```python
from build123d import *

# Parameters (mm, degrees)
SKETCH1_7_R         = 27.5
BOSS_EXTRUDE1_DEPTH = 3.5
CUT_EXTRUDE8_REACH  = 44.335
SKETCH4_R           = 6


with BuildPart() as part:
    # Sketch1 → Revolve16 (revolve)
    with BuildSketch(Plane.XY, mode=Mode.PRIVATE) as revolve16_sk:
        with BuildLine():
            Line((-9.25, 22.000000003), (-9.25, 27.485223303))
            ThreePointArc((-9.25, 27.485223303), (0, 29), (9.25, 27.485223303))
            Line((9.25, 27.485223303), (9.25, 22.000000003))
            Line((9.25, 22.000000003), (-9.25, 22.000000003))
        make_face()
    revolve(revolve16_sk.sketch.rotate(Axis((-9.25, 22.000000003, 0), (1, 0, 0)), 180), axis=Axis((-9.25, 22.000000003, 0), (1, 0, 0)))



with BuildPart() as body_2:
    # Sketch1_3 → Revolve17 (revolve)
    with BuildSketch(Plane.XY, mode=Mode.PRIVATE) as revolve17_sk:
        with BuildLine():
            Line((-18.064836163, 15.595646653), (-23.281593526, 17.29067387))
            ThreePointArc((-23.281593526, 17.29067387), (-27.580638973, 8.961492837), (-28.998407922, -0.303871681))
            Line((-28.998407922, -0.303871681), (-23.781650559, -1.998898899))
            Line((-23.781650559, -1.998898899), (-18.064836163, 15.595646653))
        make_face()
    revolve(revolve17_sk.sketch.rotate(Axis((-23.781650559, -1.998898899, 0), (0.3090169943749582, 0.9510565162951501, 0)), 180), axis=Axis((-23.781650559, -1.998898899, 0), (0.3090169943749582, 0.9510565162951501, 0)))


with BuildPart() as body_3:
    # Sketch1_4 → Revolve18 (revolve)
    with BuildSketch(Plane.XY, mode=Mode.PRIVATE) as revolve18_sk:
        with BuildLine():
            Line((-20.41468275, -12.361360295), (-23.638816111, -16.798999162))
            ThreePointArc((-23.638816111, -16.798999162), (-17.045772316, -23.461492837), (-8.672001715, -27.67302633))
            Line((-8.672001715, -27.67302633), (-5.447868354, -23.235387462))
            Line((-5.447868354, -23.235387462), (-20.41468275, -12.361360295))
        make_face()
    revolve(revolve18_sk.sketch.rotate(Axis((-5.447868354, -23.235387462, 0), (-0.8090169943749421, 0.5877852522924805, 0)), 180), axis=Axis((-5.447868354, -23.235387462, 0), (-0.8090169943749421, 0.5877852522924805, 0)))


with BuildPart() as body_4:
    # Sketch1_5 → Revolve19 (revolve)
    with BuildSketch(Plane.XY, mode=Mode.PRIVATE) as revolve19_sk:
        with BuildLine():
            Line((5.447868354, -23.235387462), (8.672001715, -27.67302633))
            ThreePointArc((8.672001715, -27.67302633), (17.045772316, -23.461492837), (23.638816111, -16.798999162))
            Line((23.638816111, -16.798999162), (20.41468275, -12.361360295))
            Line((20.41468275, -12.361360295), (5.447868354, -23.235387462))
        make_face()
    revolve(revolve19_sk.sketch.rotate(Axis((20.41468275, -12.361360295, 0), (-0.8090169943749509, -0.5877852522924685, 0)), 180), axis=Axis((20.41468275, -12.361360295, 0), (-0.8090169943749509, -0.5877852522924685, 0)))


with BuildPart() as body_5:
    # Sketch1_6 → Revolve20 (revolve)
    with BuildSketch(Plane.XY, mode=Mode.PRIVATE) as revolve20_sk:
        with BuildLine():
            Line((23.781650559, -1.998898899), (28.998407922, -0.303871681))
            ThreePointArc((28.998407922, -0.303871681), (27.580638973, 8.961492837), (23.281593526, 17.29067387))
            Line((23.281593526, 17.29067387), (18.064836163, 15.595646653))
            Line((18.064836163, 15.595646653), (23.781650559, -1.998898899))
        make_face()
    revolve(revolve20_sk.sketch.rotate(Axis((18.064836163, 15.595646653, 0), (0.30901699437494456, -0.9510565162951546, 0)), 180), axis=Axis((18.064836163, 15.595646653, 0), (0.30901699437494456, -0.9510565162951546, 0)))


with BuildPart() as part_1:
    add(part.part)

    add(body_2.part)  # Boss-Extrude1 merges body 2

    add(body_3.part)  # Boss-Extrude1 merges body 3

    add(body_4.part)  # Boss-Extrude1 merges body 4

    add(body_5.part)  # Boss-Extrude1 merges body 5
    # Sketch1_7 → Boss-Extrude1 (add, symmetric)
    with BuildSketch(Plane.XY):
        Circle(SKETCH1_7_R)
    extrude(amount=BOSS_EXTRUDE1_DEPTH, both=True)

    # Sketch4 → Cut-Extrude8 (cut, up to next)
    with BuildSketch(Plane(origin=(0, 0, -3.5), x_dir=(-1, 0, 0), z_dir=(0, 0, -1)), mode=Mode.PRIVATE) as cut_extrude8_sk1:
        Circle(SKETCH4_R)
    cut_extrude8_tool1 = extrude(cut_extrude8_sk1.sketch, amount=-CUT_EXTRUDE8_REACH, mode=Mode.PRIVATE) & part_1.part
    add(cut_extrude8_tool1.solids().sort_by_distance((0, 0, -3.5))[0], mode=Mode.SUBTRACT)


solid = part_1.part
```
Check sheet for the modelled part. Datum: model origin and axes. Units: mm. A direction names the side the tool comes from. Round coordinates to 2 decimals unless told otherwise and drop trailing zeros. Order: outer loops, then holes, each group sorted by start corner. A loop starts at its lowest first (then second) coordinate and runs counter-clockwise, first axis right, second up. Notation, with made-up numbers: (-18.75, -39.75) -> (8.25, -39.75) arc R30 ccw to (8.25, -14.75) -> close; hole circle Ø4 at (-26.5, 4). An arc over 180 degrees is marked (long way). Use CSV: the item, a comma, the result in double quotes.
(1) Material ranges on line 1 along Y through (x, z) = (-8, 4); line 2 along X through (y, z) = (-13, -4.75); line 3 along Z through (x, y) = (4, 10.5), recorded low to high. Write a range as from..to.
Worked out:
line 1,"-26.21..-14.38, 17.7..26.3"
line 2,"-20.88..-10.84, 10.84..20.88"
line 3,"-3.5..3.5"
(2) Draft check along X on faces 6 (the face through (27.78, -0.7, -0.03)), 7 (the face through (-22.063, 16.895, -0.026)), 8 (the face through (-6.5, -0.4, -3.5)), 9 (the face through (-26.19, -8.39, 0.05)). Enter one of: pulls with the +X half, pulls with the -X half, needs draft (parallel to the pull), parting line crosses it, or undercut.
Worked out:
face 6,"pulls with the +X half"
face 7,"undercut"
face 8,"undercut"
face 9,"pulls with the -X half"
(3) Depth check by flat-ended pin: pin 1 (6 mm diameter, centred on y = -20, z = -2, fed in from +X); pin 2 (8 mm diameter, centred on x = -23, y = 19, fed in from +Z); pin 3 (4 mm diameter, centred on x = 4.5, y = -10, fed in from -Z). Enter the tip coordinate at first touch or a pass-through.
Worked out:
pin 1,"x = 23.27"
pin 2,"z = 5.11"
pin 3,"z = -3.5"
(4) Tool access check on faces 1 (the face through (-22.886, -15.762, -0.026)), 2 (the face through (7.92, -26.64, -0.03)), 3 (the face through (-6.5, -0.4, 3.5)), 4 (the face through (-9.25, 26.2, 0)), 5 (the face through (9.25, 23, 4)). Record the directions out of +Z, -Z, +X, -X, +Y, -Y that give a thin tool (end or side, any length) a straight path to the whole face; none if there is none.
Worked out:
face 1,"-X"
face 2,"-Y"
face 3,"+Z"
face 4,"-X, +Y"
face 5,"+X, +Y"
(5) Cross-section at A-A (y = -7). Record the boundary of the cut face in (x, z), and give its area (3 significant figures).
Worked out:
outline,"(-26.59, -3.5) -> (26.59, -3.5) -> (26.59, 3.5) -> (-26.59, 3.5) -> close"
area,"372 mm²"
